Model file for the job. Use its own axes, mm. Face numbers are marked on the shaded views. A direction names the side the tool comes from. Round coordinates to 2 decimals unless told otherwise and drop trailing zeros. Order: outer loops, then holes, each group sorted by start corner. A loop starts at its lowest first (then second) coordinate and runs counter-clockwise, first axis right, second up. Notation, with made-up numbers: (85.5, 84.5) - (126.5, 84.5) arc R25 cw to (126.5, 98.5) - close; hole circle Ø6 at (45, 51). An arc over 180 degrees is marked (long way). Answer as CSV lines item,"result". Start each with the question number.
1. Band-saw the part on B-B on z = 15. List the corners of the cut face in (x, y), then the cut area to 3 significant figures.
2. Wall check: line 1 along Z through (x, y) = (22, 3.25); line 2 along Z through (x, y) = (1, -1.75); line 3 along Y through (x, z) = (-1.3, -15). Give the ranges that are in metal, low to high. Write a range as [from, to].
3. Pin check, flat tips, straight feed: pin 1 Ø4 at (x, z) = (17.5, 11.5) entering from -Y; pin 2 Ø1.5 at (y, z) = (-0.5, -11.5) entering from -X; pin 3 Ø3 at (x, z) = (15, 0) entering from +Y. Stop position of each tip, or through.
4. Band-saw the part on C-C on y = -8. List the corners of the cut face in (x, z), then the cut area to 3 significant figures.
5. Pull direction Z, two halves, no side cores. Call the marked faces 3 and 4: released by +Z, released by -Z, zero draft, split by the parting line, or undercut.
6. 3-axis set-ups, long thin cutter, end or side, ignore diameter. For the marked faces 1 and 2: which of +Z, -Z, +X, -X, +Y, -Y reach the whole face in a straight line?
7. Band-saw the part on D-D on z = -11. List the corners of the cut face in (x, y), then the cut area to 3 significant figures.
8. Band-saw the part on A-A on x = 15. List the corners of the cut face in (y, z).
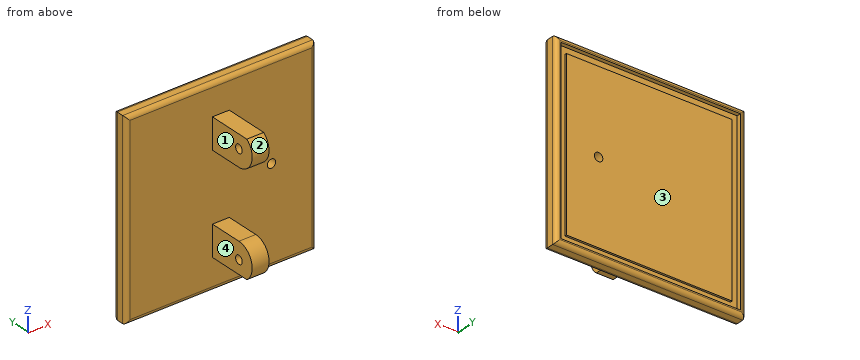
Autodesk Inventor part; units mm, degrees
ref_plane "YZ Plane" through (0, 0, 0) normal (1, 0, 0) x (0, 1, 0)
ref_plane "XZ Plane" through (0, 0, 0) normal (0, 1, 0) x (-1, 0, 0)
ref_plane "XY Plane" through (0, 0, 0) normal (0, 0, 1) x (1, 0, 0)
sketch "스케치1" plane through (0, 0, 0) normal (0, 1, 0) x (-1, 0, 0)
  line L0 (-24.9446, -24.9446) -> (24.9446, -24.9446)
  line L1 (24.9446, -24.9446) -> (24.9446, 24.9446)
  line L2 (24.9446, 24.9446) -> (-24.9446, 24.9446)
  line L3 (-24.9446, 24.9446) -> (-24.9446, -24.9446)
  line L4 (-24.9446, -24.9446) -> (24.9446, 24.9446) construction
  line L5 (24.9446, -24.9446) -> (-24.9446, 24.9446) construction
  line L6 (-28.1446, -28.1446) -> (28.1446, -28.1446)
  line L7 (28.1446, -28.1446) -> (28.1446, 28.1446)
  line L8 (28.1446, 28.1446) -> (-28.1446, 28.1446)
  line L9 (-28.1446, 28.1446) -> (-28.1446, -28.1446)
  line L10 (-28.1446, -28.1446) -> (28.1446, 28.1446) construction
  line L11 (28.1446, -28.1446) -> (-28.1446, 28.1446) construction
  point P0 (0, 0)
  dimension "d0" = 70.554
  dimension "d1" = 3.2
extrude "돌출1" add sketch "스케치1" along normal blind 4.4 contours L3 L2 L1 L0 | L9 L8 L7 L6
sketch "스케치2" plane through (0, 4.4, 0) normal (0, 1, 0) x (1, 0, 0)
  line L0 (-28.1446, 28.1446) -> (-28.1446, -28.1446)
  line L1 (-28.1446, -28.1446) -> (28.1446, -28.1446)
  line L2 (28.1446, -28.1446) -> (28.1446, 28.1446)
  line L3 (28.1446, 28.1446) -> (-28.1446, 28.1446)
  line L4 (26.5446, 26.5446) -> (-26.5446, 26.5446)
  line L5 (-26.5446, 26.5446) -> (-26.5446, -26.5446)
  line L6 (-26.5446, -26.5446) -> (26.5446, -26.5446)
  line L7 (26.5446, -26.5446) -> (26.5446, 26.5446)
  line L8 (26.5446, 26.5446) -> (-26.5446, -26.5446) construction
  line L9 (-26.5446, 26.5446) -> (26.5446, -26.5446) construction
  line L10 (24.5446, 24.5446) -> (-24.5446, 24.5446)
  line L11 (-24.5446, 24.5446) -> (-24.5446, -24.5446)
  line L12 (-24.5446, -24.5446) -> (24.5446, -24.5446)
  line L13 (24.5446, -24.5446) -> (24.5446, 24.5446)
  line L14 (24.5446, 24.5446) -> (-24.5446, -24.5446) construction
  line L15 (-24.5446, 24.5446) -> (24.5446, -24.5446) construction
  point P0 (0, 0)
  point P1 (0, 28.1446)
  point P2 (-28.1446, 0)
  dimension "d4" = 1.6
  dimension "d5" = 2
extrude "돌출2" cut sketch "스케치2" against normal blind 1.2 contours L7 L6 L5 L4 | L13 L12 L11 L10
sketch "스케치3" plane through (0, 3.2, 0) normal (0, 1, 0) x (1, 0, 0)
  line L0 (24.5446, 24.5446) -> (-24.5446, 24.5446)
  line L1 (-24.5446, 24.5446) -> (-24.5446, -24.5446)
  line L2 (-24.5446, -24.5446) -> (24.5446, -24.5446)
  line L3 (24.5446, -24.5446) -> (24.5446, 24.5446)
  line L4 (24.5446, 24.5446) -> (-24.5446, -24.5446) construction
  line L5 (-24.5446, 24.5446) -> (24.5446, -24.5446) construction
  line L6 (-26.5446, -26.5446) -> (-26.5446, 26.5446)
  point P0 (0, 0)
  dimension "d8" = 2
extrude "돌출3" add sketch "스케치3" along normal blind 0.6
fillet "모깎기1" radius 1.2 8 edges at (0, 4.4, 28.1446) (28.1446, 4.4, 0) (0, 4.4, -28.1446) (-28.1446, 4.4, 0) (-28.1446, 0, 0) (0, 0, 28.1446) (28.1446, 0, 0) (0, 0, -28.1446)
sketch "스케치6" plane through (0, 0, 0) normal (0, -1, 0) x (1, 0, 0)
  line L0 (-2.5, -20) -> (2.5, -20)
  line L1 (2.5, -20) -> (2.5, -10)
  line L2 (2.5, -10) -> (-2.5, -10)
  line L3 (-2.5, -10) -> (-2.5, -20)
  line L4 (-2.5, -20) -> (2.5, -10) construction
  line L5 (2.5, -20) -> (-2.5, -10) construction
  line L6 (-2.5, 10) -> (2.5, 10)
  line L7 (2.5, 10) -> (2.5, 20)
  line L8 (2.5, 20) -> (-2.5, 20)
  line L9 (-2.5, 20) -> (-2.5, 10)
  line L10 (-2.5, 10) -> (2.5, 20) construction
  line L11 (2.5, 10) -> (-2.5, 20) construction
  point P0 (0, 0)
  point P1 (0, -15)
  point P2 (0, 15)
  dimension "d27" = 5
  dimension "d28" = 10
  dimension "d29" = 10
  dimension "d30" = 5
  dimension "d31" = 20
  dimension "d33" = 10
extrude "돌출6" add sketch "스케치6" along normal blind 10
sketch "스케치7" plane through (2.5, 0, 20) normal (1, 0, 0) x (0, 0, -1)
  line L0 (10, -10) -> (0, -10)
  circle A0 centre (5, -10) radius 5
  line L1 (40, -10) -> (30, -10)
  circle A1 centre (35, -10) radius 5
  point P0 (20, 0)
extrude "돌출7" add sketch "스케치7" against normal blind 5
sketch "스케치8" plane through (2.5, 0, 20) normal (1, 0, 0) x (0, 0, -1)
  arc A0 (0, -10) -> (10, -10) centre (5, -10) ccw
  circle A1 centre (5, -10) radius 1.25
  arc A2 (30, -10) -> (40, -10) centre (35, -10) ccw
  circle A3 centre (35, -10) radius 1.25
  point P0 (20, 0)
  dimension "d38" = 2.5
  dimension "d39" = 2.5
extrude "돌출8" cut sketch "스케치8" against normal blind 5
sketch "스케치9" plane through (0, 0, 0) normal (0, -1, 0) x (1, 0, 0)
  line L0 (2.5, -10) -> (-2.5, -10)
  line L1 (-2.5, -20) -> (-2.5, -10)
  line L2 (-2.5, -20) -> (2.5, -20)
  line L3 (2.5, -10) -> (2.5, -20)
  line L4 (2.5, 13.75) -> (-2.5, 13.75)
  line L5 (2.5, 20) -> (-2.5, 20)
  line L6 (-2.5, 10) -> (-2.5, 20)
  line L7 (-2.5, 10) -> (2.5, 10)
  line L8 (2.5, 20) -> (2.5, 10)
  line L9 (-2.5, -19) -> (2.5, -19)
  line L10 (-2.5, 10) -> (-2.5, 20)
  line L11 (-2.5, 19) -> (2.5, 19)
  point P0 (0, 0)
  dimension "d42" = 1
  dimension "d43" = 1
extrude "돌출9" cut sketch "스케치9" along normal blind 15 contours L3 L2 L1 L9 | L11 L6 L5 L8
sketch "스케치10" plane through (0, 0, 0) normal (0, -1, 0) x (1, 0, 0)
  circle A0 centre (15, 0) radius 1.25
  point P0 (0, 0)
  dimension "d46" = 2.5
  dimension "d47" = 15
extrude "돌출10" cut sketch "스케치10" against normal blind 10
properties part number "OV-PAM_n_4_bottom"
Reply:
1,outline,"(-28.14, 1.2) arc R1.2 ccw to (-26.94, 0) - (-2.5, 0) - (-2.5, -8.75) - (2.5, -8.75) - (2.5, 0) - (26.94, 0) arc R1.2 ccw to (28.14, 1.2) - (28.14, 3.2) arc R1.2 ccw to (26.94, 4.4) - (26.54, 4.4) - (26.54, 3.2) - (24.54, 3.2) - (24.54, 3.8) - (-24.54, 3.8) - (-24.54, 3.2) - (-26.54, 3.2) - (-26.54, 4.4) - (-26.94, 4.4) arc R1.2 ccw to (-28.14, 3.2) - close; (-2.5, -15) - (2.5, -15) - (2.5, -11.25) - (-2.5, -11.25) - close"
1,area,"275 mm2"
2,line 1,"z = [-28.14, -26.54], [-24.54, 24.54], [26.54, 28.14]"
2,line 2,"z = [-19, -10], [10, 19]"
2,line 3,"y = [-15, -11.25], [-8.75, 3.8]"
3,pin 1,"stops at y = 0"
3,pin 2,"stops at x = -27.68"
3,pin 3,"stops at y = 3.8"
4,outline,"(-2.5, -19) - (2.5, -19) - (2.5, -10) - (-2.5, -10) - close; (-2.5, 10) - (2.5, 10) - (2.5, 19) - (-2.5, 19) - close"
4,area,"90.0 mm2"
5,face 3,"undercut"
5,face 4,"zero draft"
6,face 1,"+Z, -Z, -X, -Y"
6,face 2,"+X, -X, -Y"
7,outline,"(-28.14, 1.2) arc R1.2 ccw to (-26.94, 0) - (-2.5, 0) - (-2.5, -13) - (2.5, -13) - (2.5, 0) - (26.94, 0) arc R1.2 ccw to (28.14, 1.2) - (28.14, 3.2) arc R1.2 ccw to (26.94, 4.4) - (26.54, 4.4) - (26.54, 3.2) - (24.54, 3.2) - (24.54, 3.8) - (-24.54, 3.8) - (-24.54, 3.2) - (-26.54, 3.2) - (-26.54, 4.4) - (-26.94, 4.4) arc R1.2 ccw to (-28.14, 3.2) - close"
7,area,"277 mm2"
8,outline,"(0, -26.94) arc R1.2 ccw to (1.2, -28.14) - (3.2, -28.14) arc R1.2 ccw to (4.4, -26.94) - (4.4, -26.54) - (3.2, -26.54) - (3.2, -24.54) - (3.8, -24.54) - (3.8, -1.25) - (0, -1.25) - close; (0, 1.25) - (3.8, 1.25) - (3.8, 24.54) - (3.2, 24.54) - (3.2, 26.54) - (4.4, 26.54) - (4.4, 26.94) arc R1.2 ccw to (3.2, 28.14) - (1.2, 28.14) arc R1.2 ccw to (0, 26.94) - close"
